from build123d import *

# Parameters (mm, degrees)
SKETCH1_R           = 10.5
BOSS_EXTRUDE1_DEPTH = 40.5
FILLET1_R           = 3.5
SKETCH2_W           = 41.275373403
SKETCH2_H           = 50.56233242
CUT_EXTRUDE1_DEPTH  = 40.5


# Read off the part's stored shape, not the designer's step: Shell4
with BuildPart() as part:
    # Sketch1 → Boss-Extrude1 (new body)
    with BuildSketch(Plane(origin=(0, 0, 0), x_dir=(1, 0, 0), z_dir=(0, 1, 0))):
        with Locations(Location((0, 0, 0), (0, 0, 270))):
            Circle(SKETCH1_R)
    extrude(amount=BOSS_EXTRUDE1_DEPTH)

    # Fillet1
    fillet1_edges = [part.edges().sort_by_distance(p)[0] for p in [
        (0, 0, -10.5),
        (0, 40.5, -10.5),
    ]]
    fillet(fillet1_edges, radius=FILLET1_R)

    # Sketch2 → Cut-Extrude1 (cut)
    with BuildSketch(Plane(origin=(0, 0, 0), x_dir=(0, 0, -1), z_dir=(1, 0, 0))):
        with Locations((2.800828909, 23.566771077)):
            Rectangle(SKETCH2_W, SKETCH2_H)
    extrude(amount=-CUT_EXTRUDE1_DEPTH, mode=Mode.SUBTRACT)

    # Shell4 outline → Shell4 (revolve, cut)
    with BuildSketch(Plane.XY):
        with BuildLine():
            Line((0, 1), (7, 1))
            ThreePointArc((7, 1), (8.767766953, 1.732233047), (9.5, 3.5))
            Line((9.5, 3.5), (9.5, 37))
            ThreePointArc((9.5, 37), (8.767766953, 38.767766953), (7, 39.5))
            Line((7, 39.5), (7, 40.5))
            Line((7, 40.5), (0, 40.5))
            Line((0, 40.5), (0, 1))
        make_face()
    revolve(axis=Axis((0, 0, 0), (0, 1, 0)), mode=Mode.SUBTRACT)


solid = part.part
Source: CAD feature listing. Evaluate the final solid. Frame: model axes, mm. A direction names the side the tool comes from. Round coordinates to 2 decimals unless told otherwise and drop trailing zeros. Order: outer loops, then holes, each group sorted by start corner. A loop starts at its lowest first (then second) coordinate and runs counter-clockwise, first axis right, second up. Notation, with made-up numbers: (33, 34) - (60, 34) arc R28 ccw to (60, 58) - close; hole circle Ø3 at (24, 67.25). An arc over 180 degrees is marked (long way). Use a Markdown table: item, result. Add a question column.
1. Section query C-C (y = 3). Return the cut outline in (x, z).
2. Section query B-B (y = 35.5). Return the cut outline in (x, z).
3. Line query: probe 1 along Z at (x, y) = (8.5, 26); probe 2 along Z at (x, y) = (7.25, 14.5); probe 3 along Y at (x, z) = (2, 2). Output: solid intervals per line, ascending.
4. Mould query, pull axis Y, two halves, no side actions, for faces 1 (the cylindrical face through (10.5, 20, 0.2)), 2 (the flat face through (3, 1, 0)), 3 (the flat face through (3, 0, 0)), 4 (the cylindrical face through (9.498, 20.484, 0.209)). Classes: +Y half, -Y half, draft (parallel to the pull), parting line (faces both ways), or undercut.
5. Section query A-A (z = 0). Return the cut outline in (x, y), then the cut area to 3 significant figures.
6. First-contact query: pin 1 (1 mm diameter, centred on x = 6, y = 12.5, fed in from +Z); pin 2 (2 mm diameter, centred on x = 8, z = 4.5, fed in from -Y); pin 3 (1 mm diameter, centred on y = 5.5, z = -3.5, fed in from -X). Flat tips, straight axial feed; report the tip coordinate or a pass-through.
7. Set-up query: faces 5 (the cylindrical face through (7, 40, 0)), 6 (the flat face through (0, 16, 10)). Return all of +Z, -Z, +X, -X, +Y, -Y with unobstructed straight access to the full face (end or side cutting, diameter ignored); none if empty.
Derived:
| question | item | result |
|---|---|---|
| 1 | outline | (0, -10.46) arc R10.46 ccw to (0, 10.46) - (0, 9.45) arc R9.45 cw to (0, -9.45) - close |
| 2 | outline | (0, -10.5) arc R10.5 ccw to (0, 10.5) - (0, 9.5) arc R9.5 cw to (0, -9.5) - close |
| 3 | probe 1 | -6.16 to -4.24, 4.24 to 6.16 |
| 3 | probe 2 | -7.6 to -6.14, 6.14 to 7.6 |
| 3 | probe 3 | 0 to 1 |
| 4 | face 1 | draft |
| 4 | face 2 | +Y half |
| 4 | face 3 | -Y half |
| 4 | face 4 | undercut |
| 5 | outline | (0, 0) - (7, 0) arc R3.5 ccw to (10.5, 3.5) - (10.5, 37) arc R3.5 ccw to (7, 40.5) - (7, 39.5) arc R2.5 cw to (9.5, 37) - (9.5, 3.5) arc R2.5 cw to (7, 1) - (0, 1) - close |
| 5 | area | 49.9 mm2 |
| 6 | pin 1 | z = 8.94 |
| 6 | pin 2 | y = 0.2 |
| 6 | pin 3 | x = 8.62 |
| 7 | face 5 | -X, +Y |
| 7 | face 6 | +Z, -Z, -X, +Y, -Y |
